from build123d import *

# Parameters (mm, degrees)
F1_DEPTH = 28
F1_TAPER = 7
F2_DEPTH = 14
F2_TAPER = 42
F3_DEPTH = 7
F3_TAPER = 63
F4_DEPTH = 21
F4_TAPER = 14
F5_DEPTH = 14
F5_TAPER = 42


with BuildPart() as f1:
    # F0 (on Top) → F1 (new body)
    with BuildSketch(Plane.XY):
        Polygon((16.8551116583, 35), (-16.8551116583, 35), (-37.8730921145, 8.6442861301), (-30.3718617382, -24.2207515071), (0, -38.8470692461), (30.3718617382, -24.2207515071), (37.8730921145, 8.6442861301), align=None)
    extrude(amount=F1_DEPTH, taper=F1_TAPER)

    # F1_face (on face) → F2 (join)
    with BuildSketch(Plane.XY.offset(28)):
        Polygon((34.1529073262, 7.7951782287), (15.1994736711, 31.5620322947), (-15.1994736711, 31.5620322947), (-34.1529073262, 7.7951782287), (-27.3885051724, -21.8416040362), (0, -35.0312129743), (27.3885051724, -21.8416040362), align=None)
    extrude(amount=F2_DEPTH, taper=F2_TAPER)

    # F2_face (on face) → F3 (join)
    with BuildSketch(Plane.XY.offset(42)):
        Polygon((16.4497263156, -13.1182189911), (20.5124732023, 4.681838152), (9.1289093894, 18.9563756745), (-9.1289093894, 18.9563756745), (-20.5124732023, 4.681838152), (-16.4497263156, -13.1182189911), (0, -21.039989671), align=None)
    extrude(amount=F3_DEPTH, taper=F3_TAPER)

    # F0 (on Top) → F4 (join)
    with BuildSketch(Plane.XY):
        Polygon((16.8551116583, 35), (-16.8551116583, 35), (-37.8730921145, 8.6442861301), (-30.3718617382, -24.2207515071), (0, -38.8470692461), (30.3718617382, -24.2207515071), (37.8730921145, 8.6442861301), align=None)
    extrude(amount=-F4_DEPTH, taper=F4_TAPER)

    # F4_face (on face) → F5 (join)
    with BuildSketch(Plane(origin=(0, 0, -21), x_dir=(1, 0, 0), z_dir=(0, 0, -1))):
        Polygon((14.3336408618, -29.7641119403), (32.2073986635, -7.351128572), (25.8283283603, 20.5974045467), (0, 33.0356719312), (-25.8283283603, 20.5974045467), (-32.2073986635, -7.351128572), (-14.3336408618, -29.7641119403), align=None)
    extrude(amount=F5_DEPTH, taper=F5_TAPER)


solid = f1.part
Can you work these out from the model? Positions are in its coordinate system, mm. Coordinates: 2 decimals unless noted, no trailing zeros. Loops run counter-clockwise (first coordinate to the right, second up) from the corner with the lowest first, then second, coordinate; pieces in that order, holes last. Notation, with made-up numbers: (44, 18.25) - (74, 18.25) arc R34 ccw to (74, 54.25) - close; hole circle Ø7 at (10, -2). An arc over 180 degrees is marked (long way). Answer as a JSON object with one key per item and string values. Group by question number.
Item 1: If we section it at A-A (z = 15.5): List the corners of the cut face in (x, y) for me, plus the area to 3 significant figures.
Item 2: If we section it at B-B (z = 38): List the corners of the cut face in (x, y) for me.
Item 3: For pin 1 (5 mm diameter, centred on x = -17, y = -16.5, fed in from -Z); pin 2 (5 mm diameter, centred on y = -18.5, z = 22.5, fed in from -X); pin 3 (3 mm diameter, centred on x = -15, y = -25.5, fed in from -Z), each with a flat end and sliding along its axis, tell me the tip position at first contact or that it passes through.
Item 4: If I drill on L1, parallel to Y at x = -1, z = -19; L2, parallel to X at y = 10, z = -6.5; L3, parallel to Y at x = 10, z = -5.5, over which ranges is the centre line in solid material (lowest first)? Write a range as from..to.
Returned:
{
 "1": {"outline": "(-35.81, 8.17) - (-28.72, -22.9) - (0, -36.73) - (28.72, -22.9) - (35.81, 8.17) - (15.94, 33.1) - (-15.94, 33.1) - close", "area": "3,690 mm²"},
 "2": {"outline": "(-24.41, 5.57) - (-19.58, -15.61) - (0, -25.04) - (19.58, -15.61) - (24.41, 5.57) - (10.86, 22.56) - (-10.86, 22.56) - close"},
 "3": {"pin 1": "stops at z = -32.13", "pin 2": "stops at x = -29.5", "pin 3": "stops at z = -22.98"},
 "4": {"L1": "y = -33.11..30.26", "L2": "x = -34.72..34.72", "L3": "y = -32.51..33.63"}
}
